```python
from build123d import *

# Parameters (mm, degrees)
SKETCH3_W           = 19.05
SKETCH3_H           = 19.05
BOSS_EXTRUDE1_DEPTH = 19.05
SKETCH4_W           = 13.97
SKETCH4_H           = 13.97
CUT_EXTRUDE1_DEPTH  = 17.145
SKETCH5_R           = 5.08
CUT_EXTRUDE2_DEPTH  = 33.995567884


with BuildPart() as part:
    # Sketch3 → Boss-Extrude1 (new body)
    with BuildSketch(Plane.XY):
        with Locations((9.525, 9.525)):
            Rectangle(SKETCH3_W, SKETCH3_H)
    extrude(amount=BOSS_EXTRUDE1_DEPTH)

    # Sketch4 → Cut-Extrude1 (cut)
    with BuildSketch(Plane(origin=(0, 19.05, 0), x_dir=(1, 0, 0), z_dir=(0, 1, 0))):
        with Locations((9.525, -9.525)):
            Rectangle(SKETCH4_W, SKETCH4_H)
    extrude(amount=-CUT_EXTRUDE1_DEPTH, mode=Mode.SUBTRACT)

    # Sketch5 → Cut-Extrude2 (cut, through all)
    with BuildSketch(Plane(origin=(0, 0, 0), x_dir=(-1, 0, 0), z_dir=(0, -1, 0))):
        with Locations(Location((-9.525, -9.525, 0), (0, 0, 90))):
            Circle(SKETCH5_R)
    extrude(amount=-CUT_EXTRUDE2_DEPTH, mode=Mode.SUBTRACT)


solid = part.part
```
For this review, take the finished solid that the model builds, in its own axes (mm). A direction names the side the tool comes from. Round coordinates to 2 decimals unless told otherwise and drop trailing zeros. Write each loop counter-clockwise with the first axis right and the second up, starting at its lowest first coordinate (ties: lowest second). Pieces come first, ordered by that corner, then holes. Notation, with made-up numbers: M 6.25,51 L 16.25,51 A30 cw 16.25,75 Z; hole C 63.5,56 d6. An arc over 180 degrees is marked long. One line per item, written item: value. Start each with the question number.
(1) Insertion check: pin 1 (11 mm diameter, centred on y = 13.5, z = 10.5, fed in from -X); pin 2 (4 mm diameter, centred on x = 13.5, z = 10, fed in from +Y) (3 decimals). Each pin has a flat end and moves straight along its axis. Give the tip position at first contact, or say it passes through.
(2) Machinability: for faces 4 (the flat face through (0, 9, 9)), 5 (the flat face through (16.51, 11, 10)), which of the approach directions +Z, -Z, +X, -X, +Y, -Y give a long, thin tool a straight path to every point of the face, cutting with its end or side? Answer none if there is none.
(3) We need section A-A (y = 13.5). Give the boundary of the cut face in (x, z).
(4) Wall thickness on line 1 (Z direction, x = 8, y = 10); line 2 (Y direction, x = 4.5, z = 16) (3 decimals): over which ranges is each line inside the solid? List them lowest first.
(5) The part is to be moulded in two halves that separate along X. For faces 1 (the flat face through (9, 11, 2.54)), 2 (the flat face through (19.05, 9, 9)), 3 (the flat face through (14, 0, 14)), say which applies: released by +X, released by -X, zero draft, split by the parting line, or undercut.
(6) We need section D-D (z = 15.5). Give the boundary of the cut face in (x, y) (3 decimals), and give its area (3 significant figures).
(7) We need section C-C (x = 11.25). Give the boundary of the cut face in (y, z) (3 decimals), and give its area (3 significant figures).
(8) We need section B-B (z = 7.25). Give the boundary of the cut face in (x, y) (3 decimals).
Result:
1. pin 1: x = 0
1. pin 2: y = 1.905
2. face 4: +Z, -Z, -X, +Y, -Y
2. face 5: +Y
3. outline: M 0,0 L 19.05,0 L 19.05,19.05 L 0,19.05 Z; hole M 2.54,2.54 L 16.51,2.54 L 16.51,16.51 L 2.54,16.51 Z
4. line 1: 0 to 2.54, 16.51 to 19.05
4. line 2: 0 to 1.905
5. face 1: undercut
5. face 2: released by +X
5. face 3: zero draft
6. outline: M 0,0 L 19.05,0 L 19.05,19.05 L 16.51,19.05 L 16.51,1.905 L 2.54,1.905 L 2.54,19.05 L 0,19.05 Z
6. area: 123 mm²
7. outline: M 0,0 L 19.05,0 L 19.05,2.54 L 1.905,2.54 L 1.905,4.747 L 0,4.747 Z; M 0,14.303 L 1.905,14.303 L 1.905,16.51 L 19.05,16.51 L 19.05,19.05 L 0,19.05 Z
7. area: 105 mm²
8. outline: M 0,0 L 4.983,0 L 4.983,1.905 L 2.54,1.905 L 2.54,19.05 L 0,19.05 Z; M 14.067,0 L 19.05,0 L 19.05,19.05 L 16.51,19.05 L 16.51,1.905 L 14.067,1.905 Z
